```python
from build123d import *

# Parameters (mm, degrees)
SKETCH1_W           = 138.6
SKETCH1_H           = 70.5
SKETCH1_W_2         = 128.6
SKETCH1_H_2         = 32.5
BOSS_EXTRUDE1_DEPTH = 20
SKETCH2_W           = 129.6
SKETCH2_H           = 62
CUT_EXTRUDE1_DEPTH  = 17
FILLET2_R           = 5
FILLET3_R           = 2
SKETCH3_W           = 4.5
SKETCH3_H           = 12
CUT_EXTRUDE2_DEPTH  = 14
BOSS_EXTRUDE2_DEPTH = 2


with BuildPart() as part:
    # Sketch1 → Boss-Extrude1 (new body)
    with BuildSketch(Plane.XY):
        with Locations((-15.947491639, 11.815217391)):
            Rectangle(SKETCH1_W, SKETCH1_H)
        with Locations((-15.947491639, 25.815217391)):
            Rectangle(SKETCH1_W_2, SKETCH1_H_2, mode=Mode.SUBTRACT)
    extrude(amount=BOSS_EXTRUDE1_DEPTH)

    # Sketch2 → Cut-Extrude1 (cut)
    with BuildSketch(Plane.XY.offset(20)):
        with Locations((-15.947491639, 11.565217391)):
            Rectangle(SKETCH2_W, SKETCH2_H)
    extrude(amount=-CUT_EXTRUDE1_DEPTH, mode=Mode.SUBTRACT)

    # Fillet2
    fillet2_edges = [part.edges().sort_by_distance(p)[0] for p in [
        (-85.247491639, 47.065217391, 10),
        (53.352508361, 47.065217391, 10),
        (53.352508361, -23.434782609, 10),
        (-85.247491639, -23.434782609, 10),
    ]]
    fillet(fillet2_edges, radius=FILLET2_R)

    # Fillet3
    fillet3_edges = [part.edges().sort_by_distance(p)[0] for p in [
        (-15.947491639, 47.065217391, 0),
        (-85.247491639, 11.815217391, 0),
        (53.352508361, 11.815217391, 0),
        (-15.947491639, -23.434782609, 0),
        (51.888042267, -21.970316515, 0),
        (-83.783025545, -21.970316515, 0),
        (-83.783025545, 45.600751297, 0),
        (51.888042267, 45.600751297, 0),
    ]]
    fillet(fillet3_edges, radius=FILLET3_R)

    # Sketch3 → Cut-Extrude2 (cut)
    with BuildSketch(Plane.XY.offset(20)):
        with Locations((51.102508361, -5.434782609)):
            Rectangle(SKETCH3_W, SKETCH3_H)
    extrude(amount=-CUT_EXTRUDE2_DEPTH, mode=Mode.SUBTRACT)

    # Sketch4 → Boss-Extrude2 (add)
    with BuildSketch(Plane.XY.offset(20)):
        Polygon((-60.747491639, 42.565217391), (-80.747491639, 22.565217391), (-80.747491639, 42.565217391), align=None)
        Polygon((48.852508361, 22.565217391), (48.852508361, 42.565217391), (28.852508361, 42.565217391), align=None)
    extrude(amount=-BOSS_EXTRUDE2_DEPTH)


solid = part.part
```
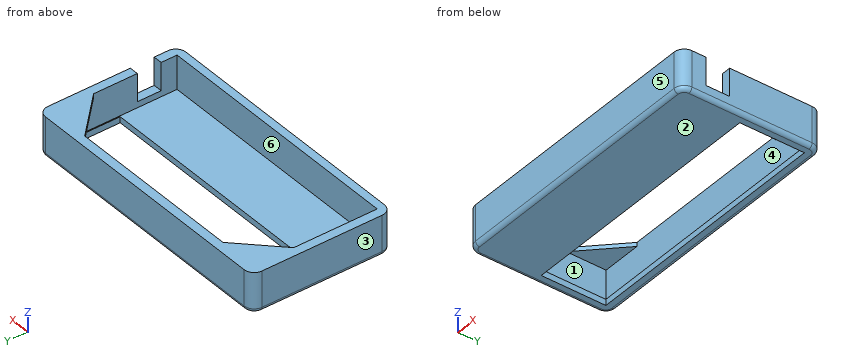
Source: CAD feature listing. Evaluate the final solid. Frame: model axes, mm. Face numbers are marked on the shaded views. A direction names the side the tool comes from. Give positions to 0.01 mm unless a question says otherwise; leave off trailing zeros. Order: outer loops, then holes, each group sorted by start corner. A loop starts at its lowest first (then second) coordinate and runs counter-clockwise, first axis right, second up.
(1) Access query for the marked faces 4, 5 and 6. Directions: +Z, -Z, +X, -X, +Y, -Y. A direction counts if a zero-diameter tool reaches every point of the face in a straight line with its end or side. Return the directions, or none.
(2) Pull-direction query (Z, two-part tool) for the marked faces 1, 2 and 3; classes: +Z half, -Z half, draft (parallel to the pull), parting line (faces both ways), or undercut.
(3) Contact query for flat-ended pins moving along their axis: P1, Ø3.5, axis at x = 50.5, z = 14, coming from the +Y side; P2, Ø2, axis at x = 50, y = -6, coming from the +Z side; P3, Ø12, axis at x = -59, y = -13, coming from the +Z side. Output: stop coordinate, or through.
(4) Section query C-C (y = -6). Return the cut outline in (x, z), plus the area to 3 significant figures.
(5) Material intervals for line 1 along Y through (x, z) = (-59.5, 13.75); line 2 along X through (y, z) = (6.5, 4); line 3 along Y through (x, z) = (25, 1.75), sorted ascending.
(6) Section query B-B (y = 34.5). Return the cut outline in (x, z).
(7) Section query A-A (x = -42.5). Return the cut outline in (y, z), plus the area to 3 significant figures.
(8) Section query D-D (z = 8.5). Return the cut outline in (x, y), plus the area to 3 significant figures.
Outcome:
1. face 4: none
1. face 5: +Z, -Z, +X, -X, -Y
1. face 6: +Z
2. face 1: undercut
2. face 2: -Z half
2. face 3: draft
3. P1: stops at y = 47.05
3. P2: stops at z = 6
3. P3: stops at z = 3
4. outline: (-85.25, 2) arc R2 ccw to (-83.25, 0) - (51.35, 0) arc R2 ccw to (53.35, 2) - (53.35, 6) - (48.85, 6) - (48.85, 3) - (-80.75, 3) - (-80.75, 20) - (-85.25, 20) - close
4. area: 504 mm2
5. line 1: y = -23.43 to -19.43, 42.57 to 47.07
5. line 2: x = -85.25 to -80.75, 48.85 to 53.35
5. line 3: y = -23.42 to 9.57, 42.07 to 47.05
6. outline: (-85.25, 2) arc R2 ccw to (-83.25, 0) - (-80.25, 0) - (-80.25, 3) - (-80.75, 3) - (-80.75, 18) - (-68.81, 18) - (-68.81, 20) - (-85.25, 20) - close; (36.92, 18) - (48.85, 18) - (48.85, 3) - (48.35, 3) - (48.35, 0) - (51.35, 0) arc R2 ccw to (53.35, 2) - (53.35, 20) - (36.92, 20) - close
7. outline: (-23.43, 2) arc R2 ccw to (-21.43, 0) - (9.57, 0) - (9.57, 3) - (-19.43, 3) - (-19.43, 20) - (-23.43, 20) - close; (42.07, 0) - (45.07, 0) arc R2 ccw to (47.07, 2) - (47.07, 20) - (42.57, 20) - (42.57, 3) - (42.07, 3) - close
7. area: 257 mm2
8. outline: (-85.25, -18.43) arc R5 ccw to (-80.25, -23.43) - (48.35, -23.43) arc R5 ccw to (53.35, -18.43) - (53.35, -11.43) - (48.85, -11.43) - (48.85, -19.43) - (-80.75, -19.43) - (-80.75, 42.57) - (48.85, 42.57) - (48.85, 0.57) - (53.35, 0.57) - (53.35, 42.07) arc R5 ccw to (48.35, 47.07) - (-80.25, 47.07) arc R5 ccw to (-85.25, 42.07) - close
8. area: 1,660 mm2
